```python
from build123d import *

# Parameters (mm, degrees)
MODEL_R             = 1.775
MODEL_R_2           = 5.5
MODEL_R_3           = 2
MODEL_R_4           = 5.125
BOSS_EXTRUDE1_DEPTH = 6.6


with BuildPart() as part:
    # Model → Boss-Extrude1 (new body)
    with BuildSketch(Plane.XY):
        with BuildLine():
            Line((40.15, 110.14), (40.15, 106.14))
            ThreePointArc((40.15, 106.14), (40.882233047, 104.372233047), (42.65, 103.64))
            Line((42.65, 103.64), (52.65, 103.64))
            ThreePointArc((52.65, 103.64), (54.417766953, 104.372233047), (55.15, 106.14))
            Line((55.15, 106.14), (55.15, 110.14))
            Line((55.15, 110.14), (79.05, 110.14))
            Line((79.05, 110.14), (79.05, 121.14))
            Line((79.05, 121.14), (77.465, 121.14))
            ThreePointArc((77.465, 121.14), (77.111446609, 121.286446609), (76.965, 121.64))
            Line((76.965, 121.64), (76.965, 125.64))
            ThreePointArc((76.965, 125.64), (77.111446609, 125.993553391), (77.465, 126.14))
            Line((77.465, 126.14), (79.05, 126.14))
            Line((79.05, 126.14), (79.05, 130.64))
            ThreePointArc((79.05, 130.64), (79.196446609, 130.993553391), (79.55, 131.14))
            Line((79.55, 131.14), (82.1, 131.14))
            ThreePointArc((82.1, 131.14), (82.453553391, 130.993553391), (82.6, 130.64))
            Line((82.6, 130.64), (82.6, 126.14))
            Line((82.6, 126.14), (84.185, 126.14))
            ThreePointArc((84.185, 126.14), (84.538553391, 125.993553391), (84.685, 125.64))
            Line((84.685, 125.64), (84.685, 121.64))
            ThreePointArc((84.685, 121.64), (84.538553391, 121.286446609), (84.185, 121.14))
            Line((84.185, 121.14), (82.6, 121.14))
            Line((82.6, 121.14), (82.6, 110.14))
            Line((82.6, 110.14), (95.3, 110.14))
            Line((95.3, 110.14), (95.3, 20))
            Line((95.3, 20), (115.3, 0))
            Line((115.3, 0), (349.1, 0))
            Line((349.1, 0), (369.1, 20))
            Line((369.1, 20), (369.1, 328.72))
            Line((369.1, 328.72), (349.1, 348.72))
            Line((349.1, 348.72), (116.05, 348.72))
            Line((116.05, 348.72), (96.05, 328.72))
            Line((96.05, 328.72), (96.05, 297.92))
            Line((96.05, 297.92), (82.6, 297.92))
            Line((82.6, 297.92), (82.6, 286.92))
            Line((82.6, 286.92), (84.185, 286.92))
            ThreePointArc((84.185, 286.92), (84.538553391, 286.773553391), (84.685, 286.42))
            Line((84.685, 286.42), (84.685, 282.42))
            ThreePointArc((84.685, 282.42), (84.538553391, 282.066446609), (84.185, 281.92))
            Line((84.185, 281.92), (82.6, 281.92))
            Line((82.6, 281.92), (82.6, 277.42))
            ThreePointArc((82.6, 277.42), (82.453553391, 277.066446609), (82.1, 276.92))
            Line((82.1, 276.92), (79.55, 276.92))
            ThreePointArc((79.55, 276.92), (79.196446609, 277.066446609), (79.05, 277.42))
            Line((79.05, 277.42), (79.05, 281.92))
            Line((79.05, 281.92), (77.465, 281.92))
            ThreePointArc((77.465, 281.92), (77.111446609, 282.066446609), (76.965, 282.42))
            Line((76.965, 282.42), (76.965, 286.42))
            ThreePointArc((76.965, 286.42), (77.111446609, 286.773553391), (77.465, 286.92))
            Line((77.465, 286.92), (79.05, 286.92))
            Line((79.05, 286.92), (79.05, 297.92))
            Line((79.05, 297.92), (55.15, 297.92))
            Line((55.15, 297.92), (55.15, 301.92))
            ThreePointArc((55.15, 301.92), (54.417766953, 303.687766953), (52.65, 304.42))
            Line((52.65, 304.42), (42.65, 304.42))
            ThreePointArc((42.65, 304.42), (40.882233047, 303.687766953), (40.15, 301.92))
            Line((40.15, 301.92), (40.15, 297.92))
            Line((40.15, 297.92), (26.41, 297.92))
            Line((26.41, 297.92), (26.41, 286.92))
            Line((26.41, 286.92), (27.995, 286.92))
            ThreePointArc((27.995, 286.92), (28.348553391, 286.773553391), (28.495, 286.42))
            Line((28.495, 286.42), (28.495, 282.42))
            ThreePointArc((28.495, 282.42), (28.348553391, 282.066446609), (27.995, 281.92))
            Line((27.995, 281.92), (26.41, 281.92))
            Line((26.41, 281.92), (26.41, 277.42))
            ThreePointArc((26.41, 277.42), (26.263553391, 277.066446609), (25.91, 276.92))
            Line((25.91, 276.92), (23.36, 276.92))
            ThreePointArc((23.36, 276.92), (23.006446609, 277.066446609), (22.86, 277.42))
            Line((22.86, 277.42), (22.86, 281.92))
            Line((22.86, 281.92), (21.275, 281.92))
            ThreePointArc((21.275, 281.92), (20.921446609, 282.066446609), (20.775, 282.42))
            Line((20.775, 282.42), (20.775, 286.42))
            ThreePointArc((20.775, 286.42), (20.921446609, 286.773553391), (21.275, 286.92))
            Line((21.275, 286.92), (22.86, 286.92))
            Line((22.86, 286.92), (22.86, 297.92))
            Line((22.86, 297.92), (2, 297.92))
            Line((2, 297.92), (0, 295.92))
            Line((0, 295.92), (0, 112.14))
            Line((0, 112.14), (2, 110.14))
            Line((2, 110.14), (22.86, 110.14))
            Line((22.86, 110.14), (22.86, 121.14))
            Line((22.86, 121.14), (21.275, 121.14))
            ThreePointArc((21.275, 121.14), (20.921446609, 121.286446609), (20.775, 121.64))
            Line((20.775, 121.64), (20.775, 125.64))
            ThreePointArc((20.775, 125.64), (20.921446609, 125.993553391), (21.275, 126.14))
            Line((21.275, 126.14), (22.86, 126.14))
            Line((22.86, 126.14), (22.86, 130.64))
            ThreePointArc((22.86, 130.64), (23.006446609, 130.993553391), (23.36, 131.14))
            Line((23.36, 131.14), (25.91, 131.14))
            ThreePointArc((25.91, 131.14), (26.263553391, 130.993553391), (26.41, 130.64))
            Line((26.41, 130.64), (26.41, 126.14))
            Line((26.41, 126.14), (27.995, 126.14))
            ThreePointArc((27.995, 126.14), (28.348553391, 125.993553391), (28.495, 125.64))
            Line((28.495, 125.64), (28.495, 121.64))
            ThreePointArc((28.495, 121.64), (28.348553391, 121.286446609), (27.995, 121.14))
            Line((27.995, 121.14), (26.41, 121.14))
            Line((26.41, 121.14), (26.41, 110.14))
            Line((26.41, 110.14), (40.15, 110.14))
        make_face()
        with Locations((123.225, 301.35)):
            Circle(MODEL_R, mode=Mode.SUBTRACT)
        with Locations((196.975, 301.35)):
            Circle(MODEL_R, mode=Mode.SUBTRACT)
        with Locations((123.225, 106.69)):
            Circle(MODEL_R, mode=Mode.SUBTRACT)
        with Locations((196.975, 106.69)):
            Circle(MODEL_R, mode=Mode.SUBTRACT)
        with Locations((120.924806781, 249.972001664)):
            Circle(MODEL_R_2, mode=Mode.SUBTRACT)
        with Locations((17.84, 185.23)):
            Circle(MODEL_R, mode=Mode.SUBTRACT)
        with Locations((45.79, 185.23)):
            Circle(MODEL_R, mode=Mode.SUBTRACT)
        with Locations((61.09, 237.62)):
            Circle(MODEL_R, mode=Mode.SUBTRACT)
        with Locations((12.84, 237.62)):
            Circle(MODEL_R, mode=Mode.SUBTRACT)
        with Locations((14.175, 172.42)):
            Circle(MODEL_R, mode=Mode.SUBTRACT)
        with Locations((75.175, 172.42)):
            Circle(MODEL_R, mode=Mode.SUBTRACT)
        with Locations((14.175, 267.42)):
            Circle(MODEL_R, mode=Mode.SUBTRACT)
        with Locations((75.175, 267.42)):
            Circle(MODEL_R, mode=Mode.SUBTRACT)
        with Locations((71.3, 292.92)):
            Circle(MODEL_R_3, mode=Mode.SUBTRACT)
        with Locations((71.3, 115.14)):
            Circle(MODEL_R_3, mode=Mode.SUBTRACT)
        with Locations((307.1, 312.72)):
            Circle(MODEL_R_4, mode=Mode.SUBTRACT)
        with Locations((118.629064244, 154.525625)):
            Circle(MODEL_R_4, mode=Mode.SUBTRACT)
        with Locations((307.1, 42.845)):
            Circle(MODEL_R_4, mode=Mode.SUBTRACT)
    extrude(amount=BOSS_EXTRUDE1_DEPTH)


solid = part.part
```
Work out the finished part from the listing and answer in its coordinate system (mm). Round coordinates to 2 decimals unless told otherwise and drop trailing zeros. Loops run counter-clockwise (first coordinate to the right, second up) from the corner with the lowest first, then second, coordinate; pieces in that order, holes last.
(1) The part is cut by section B-B, the plane z = 2.75. Give the number of separate pieces and of enclosed holes in the cut face, and give its area (3 significant figures).
Computed values:
separate pieces: 1
enclosed holes: 18
area: 112,000 mm2
(2) Find the intervals of material crossed by L1, parallel to X at y = 237.62, z = 3.25 (3 decimals); L2, parallel to Y at x = 71.3, z = 4.75; L3, parallel to X at y = 281, z = 4.75, in increasing order.
Computed values:
L1: x = 0 to 11.065, 14.615 to 59.315, 62.865 to 369.1
L2: y = 110.14 to 113.14, 117.14 to 290.92, 294.92 to 297.92
L3: x = 0 to 22.86, 26.41 to 79.05, 82.6 to 369.1
(3) Each of these flat-tipped pins is pushed along its axis until it touches: P1, Ø0.5, axis at x = 83.5, z = 3, coming from the -Y side; P2, Ø3.5, axis at x = 30, z = 2, coming from the +Y side; P3, Ø3.5, axis at x = 47, z = 4.5, coming from the +Y side. Where does it stop, or does it pass through?
Computed values:
P1: stops at y = 110.14
P2: stops at y = 297.92
P3: stops at y = 304.42
(4) The part is cut by section A-A, the plane y = 312.72. Give the vertices of the cut face in (x, z) (3 decimals), and give its area (3 significant figures).
Computed values:
outline: (96.05, 0) - (301.975, 0) - (301.975, 6.6) - (96.05, 6.6) - close; (312.225, 0) - (369.1, 0) - (369.1, 6.6) - (312.225, 6.6) - close
area: 1,730 mm2
(5) The mould has two halves that part along Y. Classify faces 1 (the flat face through (359.24, 338.58, 3.25)), 2 (the cylindrical face through (123.46, 245.09, 3.25)), 3 (the flat face through (182, 177, 6.6)), 4 (the cylindrical face through (303.03, 39.73, 3.25)): pulls with the +Y half, pulls with the -Y half, needs draft (parallel to the pull), parting line crosses it, or undercut.
Computed values:
face 1: pulls with the +Y half
face 2: undercut
face 3: needs draft
face 4: undercut
